Can you work these out from the model? Positions are in its coordinate system, mm. A direction names the side the tool comes from. Give positions to 0.01 mm unless a question says otherwise; leave off trailing zeros. Order: outer loops, then holes, each group sorted by start corner. A loop starts at its lowest first (then second) coordinate and runs counter-clockwise, first axis right, second up. Notation, with made-up numbers: M 45.25,64.25 L 53.25,64.25 A27 cw 53.25,87.25 Z; hole C 52,28.25 d4. An arc over 180 degrees is marked long. Answer as a JSON object with one key per item and string values.
```python
from build123d import *

# Parameters (mm, degrees)
BOSS_EXTRUDE1_DEPTH = 2.5
SKETCH4_R           = 0.35
THROUGH_HOLES_DEPTH = 7.493265742
FILLET1_R           = 0.125
SKETCH5_R           = 0.125
BOSS_EXTRUDE2_DEPTH = 0.5


with BuildPart() as part:
    # Sketch3 → Boss-Extrude1 (new body)
    with BuildSketch(Plane(origin=(0, 0, 0), x_dir=(1, 0, 0), z_dir=(0, 1, 0))):
        with BuildLine():
            Line((-2.5, 0.9), (-2, 0.93))
            Line((-2, 0.93), (-2, 0.56))
            Line((-2, 0.56), (-1.5, 0.56))
            Line((-1.5, 0.56), (-1.5, 0.96))
            Line((-1.5, 0.96), (0, 1.05))
            ThreePointArc((0, 1.05), (1.05, 0), (0, -1.05))
            Line((0, -1.05), (-1.5, -0.96))
            Line((-1.5, -0.96), (-1.5, -0.56))
            Line((-1.5, -0.56), (-2, -0.56))
            Line((-2, -0.56), (-2, -0.93))
            Line((-2, -0.93), (-2.5, -0.9))
            Line((-2.5, -0.9), (-5, -0.9))
            ThreePointArc((-5, -0.9), (-5.9, 0), (-5, 0.9))
            Line((-5, 0.9), (-2.5, 0.9))
        make_face()
    extrude(amount=BOSS_EXTRUDE1_DEPTH)

    # Sketch4 → Through Holes (cut, through all)
    with BuildSketch(Plane(origin=(0, 2.5, 0), x_dir=(1, 0, 0), z_dir=(0, 1, 0))):
        with BuildLine():
            Line((-4.1375, 0.9), (-4.7125, 0.9))
            Line((-4.7125, 0.9), (-4.7125, 0.2875))
            Line((-4.7125, 0.2875), (-5, 0.2875))
            ThreePointArc((-5, 0.2875), (-5.2875, 0), (-5, -0.2875))
            Line((-5, -0.2875), (-4.1375, -0.2875))
            Line((-4.1375, -0.2875), (-4.1375, 0.9))
        make_face()
        with Locations(Location((0, 0, 0), (0, 0, 270))):
            Circle(SKETCH4_R)
    extrude(amount=-THROUGH_HOLES_DEPTH, mode=Mode.SUBTRACT)

    # Fillet1
    fillet1_edges = [part.edges().sort_by_distance(p)[0] for p in [
        (-2, 1.25, 0.56),
        (-1.5, 1.25, 0.56),
        (-1.5, 1.25, -0.56),
        (-2, 1.25, -0.56),
        (-4.7125, 1.25, -0.9),
        (-4.1375, 1.25, -0.9),
    ]]
    fillet(fillet1_edges, radius=FILLET1_R)

    # Sketch5 → Boss-Extrude2 (add)
    with BuildSketch(Plane(origin=(0, 0, 0), x_dir=(1, 0, 0), z_dir=(0, 1, 0))):
        with BuildLine():
            Line((-1.514973073, -1.209551211), (-1.514973073, 1.209551211))
            Line((-1.514973073, 1.209551211), (-0.007892579, 1.299976041))
            ThreePointArc((-0.007892579, 1.299976041), (1.3, 0), (-0.007892579, -1.299976041))
            Line((-0.007892579, -1.299976041), (-1.514973073, -1.209551211))
        make_face()
        with Locations(Location((0, 0, 0), (0, 0, 270))):
            Circle(SKETCH5_R, mode=Mode.SUBTRACT)
    extrude(amount=-BOSS_EXTRUDE2_DEPTH)


solid = part.part
```
1) I need wall thicknesses on L1, parallel to X at y = 1.25, z = 0; L2, parallel to X at y = 1.95, z = -0.8; L3, parallel to Y at x = -3.25, z = 0. Which ranges of each line are inside material? Lowest first, please.
Results found:
{"L1": "x = -5.9 to -5.29, -4.14 to -0.35, 0.35 to 1.05", "L2": "x = -5.41 to -4.72, -4.13 to -2, -1.5 to 0.68", "L3": "y = 0 to 2.5"}
2) Thinking about a two-plate mould opening in Z: for faces 1 (the face through (-4.6, 1.3, 0.288)), 2 (the face through (-3.7, 0, 0)), 3 (the face through (-5.9, 1.2, 0)), which applies, pulls with the +Z half, pulls with the -Z half, needs draft (parallel to the pull), parting line crosses it, or undercut?
Results found:
{"face 1": "undercut", "face 2": "needs draft", "face 3": "parting line crosses it"}
3) I'm going to push flat-ended pins straight in: pin 1 Ø1.5 at (x, z) = (-4, 0) entering from -Y; pin 2 Ø1.5 at (y, z) = (1.5, -1) entering from +X; pin 3 Ø0.8 at (x, z) = (0, 0) entering from +Y; pin 4 Ø0.8 at (x, y) = (-3, 1) entering from -Z. Where does each tip first touch, or does it pass through?
Results found:
{"pin 1": "stops at y = 0", "pin 2": "stops at x = 1.02", "pin 3": "stops at y = 2.5", "pin 4": "stops at z = -0.9"}
4) For faces 4 (the face through (-4.138, 1, 0)), 5 (the face through (-0.74, 1.232, 1.006)), 6 (the face through (-4, 1, 0.9)), 7 (the face through (-3, 1, -0.9)), which set-ups out of +Z, -Z, +X, -X, +Y, -Y let a thin tool reach every point of the face, with its end or its side?
Results found:
{"face 4": "-Z, +Y, -Y", "face 5": "+Z, -X, +Y", "face 6": "+Z, -X, +Y, -Y", "face 7": "-Z, -X, +Y, -Y"}
5) I want a section at D-D on z = 0.45. Write out the boundary of the cut face in (x, y).
Results found:
{"outline": "M -5.78,0 L -1.51,0 L -1.51,-0.5 L 1.22,-0.5 L 1.22,0 L 0.95,0 L 0.95,2.5 L -5.78,2.5 Z"}
6) I want a section at C-C on x = -3. Write out the boundary of the cut face in (y, z).
Results found:
{"outline": "M 0,-0.9 L 2.5,-0.9 L 2.5,0.9 L 0,0.9 Z"}
7) I want a section at A-A on z = 0. Count the separate pieces of the cut face and the enclosed holes in it, and give its area (3 significant figures).
Results found:
{"separate pieces": "3", "enclosed holes": "0", "area": "14.0 mm²"}
